For this review, take the finished solid that the model builds, in its own axes (mm). Coordinates: 2 decimals unless noted, no trailing zeros. Loops run counter-clockwise (first coordinate to the right, second up) from the corner with the lowest first, then second, coordinate; pieces in that order, holes last. Notation, with made-up numbers: (-21, 40.5) - (19, 40.5) arc R23 ccw to (19, 59.5) - close; hole circle Ø5 at (27.25, -7.75). An arc over 180 degrees is marked (long way). One line per item, written item: value. Start each with the question number.
1. Take a section at B-B, the plane y = 645.5. State the section outline as (x, z) points, and give its area (3 significant figures).
2. Take a section at A-A, the plane x = 1089.5. State the section outline as (y, z) points, and give its area (3 significant figures).
3. To check wall thickness, follow line 1 (Y direction, x = 1092.5, z = 1.15); line 2 (Y direction, x = 1080.5, z = 0.65); line 3 (X direction, y = 657, z = 0.2). State the ranges of each line that lie inside material, in increasing order. Write a range as from..to.
4. Insertion check: pin 1 (1 mm diameter, centred on x = 1094, z = 0.5, fed in from -Y); pin 2 (0.6 mm diameter, centred on x = 1091.5, z = 1, fed in from -Y); pin 3 (0.6 mm diameter, centred on y = 678, z = 1.5, fed in from +X). Each pin has a flat end and moves straight along its axis. Give the tip position at first contact, or say it passes through.
```python
from build123d import *

# Parameters (mm, degrees)
EXTRUDE_1_DEPTH = 2


with BuildPart() as part:
    # Model → 凸台-拉伸1 (new body)
    with BuildSketch(Plane.XY):
        Polygon((1047.912570376, 680.457705055), (1047.912570376, 676.068532902), (1052.912570376, 676.068532902), (1052.912570376, 671.068532902), (1047.912570376, 671.068532902), (1047.912570376, 668.573157352), (1045.412570376, 668.573157352), (1045.412570376, 658.573157352), (1047.912570376, 658.573157352), (1047.912570376, 643.128332902), (1046.412570376, 643.128332902), (1046.412570376, 633.128332902), (1047.912570376, 633.128332902), (1047.912570376, 629.068532902), (1052.912570376, 629.068532902), (1052.912570376, 624.068532902), (1057.912570376, 624.068532902), (1057.912570376, 623.068532902), (1067.912570376, 623.068532902), (1067.912570376, 624.068532902), (1072.912570376, 624.068532902), (1072.912570376, 623.068532902), (1082.912570376, 623.068532902), (1082.912570376, 624.068532902), (1087.912570376, 624.068532902), (1087.912570376, 629.068532902), (1092.912570376, 629.068532902), (1092.912570376, 633.128332902), (1094.412570376, 633.128332902), (1094.412570376, 643.128332902), (1092.912570376, 643.128332902), (1092.912570376, 658.573157352), (1095.412570376, 658.573157352), (1095.412570376, 668.573157352), (1092.912570376, 668.573157352), (1092.912570376, 671.068532902), (1087.912570376, 671.068532902), (1087.912570376, 676.068532902), (1092.912570376, 676.068532902), (1092.912570376, 680.457705055), align=None)
        with BuildLine():
            Line((1057.912570376, 668.068532902), (1057.912570376, 673.218532902))
            ThreePointArc((1057.912570376, 673.218532902), (1057.440095607, 674.509527351), (1056.245903709, 675.190559496))
            ThreePointArc((1056.245903709, 675.190559496), (1055.64880776, 675.531075569), (1055.412570376, 676.176572793))
            Line((1055.412570376, 676.176572793), (1055.412570376, 676.867577668))
            ThreePointArc((1055.412570376, 676.867577668), (1055.705463595, 677.57468445), (1056.412570376, 677.867577668))
            Line((1056.412570376, 677.867577668), (1083.912570376, 677.867577668))
            ThreePointArc((1083.912570376, 677.867577668), (1084.619677157, 677.57468445), (1084.912570376, 676.867577668))
            Line((1084.912570376, 676.867577668), (1084.912570376, 676.046960027))
            ThreePointArc((1084.912570376, 676.046960027), (1084.729066957, 675.469609757), (1084.245903709, 675.104150985))
            ThreePointArc((1084.245903709, 675.104150985), (1083.279577214, 674.37323344), (1082.912570376, 673.218532902))
            Line((1082.912570376, 673.218532902), (1082.912570376, 668.068532902))
            ThreePointArc((1082.912570376, 668.068532902), (1083.498356813, 666.65431934), (1084.912570376, 666.068532902))
            Line((1084.912570376, 666.068532902), (1085.912570376, 666.068532902))
            ThreePointArc((1085.912570376, 666.068532902), (1087.326783938, 665.482746464), (1087.912570376, 664.068532902))
            Line((1087.912570376, 664.068532902), (1087.912570376, 636.068532902))
            ThreePointArc((1087.912570376, 636.068532902), (1087.326783938, 634.65431934), (1085.912570376, 634.068532902))
            Line((1085.912570376, 634.068532902), (1084.912570376, 634.068532902))
            ThreePointArc((1084.912570376, 634.068532902), (1083.498356813, 633.482746464), (1082.912570376, 632.068532902))
            Line((1082.912570376, 632.068532902), (1082.912570376, 631.068532902))
            ThreePointArc((1082.912570376, 631.068532902), (1082.326783938, 629.65431934), (1080.912570376, 629.068532902))
            Line((1080.912570376, 629.068532902), (1059.912570376, 629.068532902))
            ThreePointArc((1059.912570376, 629.068532902), (1058.498356813, 629.65431934), (1057.912570376, 631.068532902))
            Line((1057.912570376, 631.068532902), (1057.912570376, 632.068532902))
            ThreePointArc((1057.912570376, 632.068532902), (1057.326783938, 633.482746464), (1055.912570376, 634.068532902))
            Line((1055.912570376, 634.068532902), (1054.912570376, 634.068532902))
            ThreePointArc((1054.912570376, 634.068532902), (1053.498356813, 634.65431934), (1052.912570376, 636.068532902))
            Line((1052.912570376, 636.068532902), (1052.912570376, 664.068532902))
            ThreePointArc((1052.912570376, 664.068532902), (1053.498356813, 665.482746464), (1054.912570376, 666.068532902))
            Line((1054.912570376, 666.068532902), (1055.912570376, 666.068532902))
            ThreePointArc((1055.912570376, 666.068532902), (1057.326783938, 666.65431934), (1057.912570376, 668.068532902))
        make_face(mode=Mode.SUBTRACT)
    extrude(amount=EXTRUDE_1_DEPTH)


solid = part.part
```
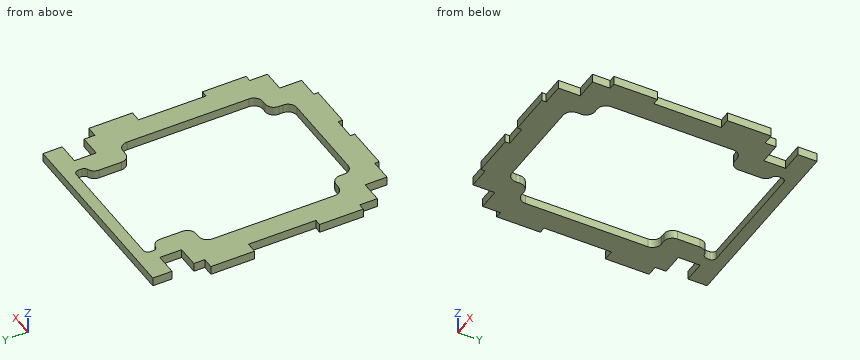
Solutions:
1. outline: (1047.91, 0) - (1052.91, 0) - (1052.91, 2) - (1047.91, 2) - close; (1087.91, 0) - (1092.91, 0) - (1092.91, 2) - (1087.91, 2) - close
1. area: 20.0 mm2
2. outline: (629.07, 0) - (671.07, 0) - (671.07, 2) - (629.07, 2) - close; (676.07, 0) - (680.46, 0) - (680.46, 2) - (676.07, 2) - close
2. area: 92.8 mm2
3. line 1: 629.07..671.07, 676.07..680.46
3. line 2: 623.07..629.07, 677.87..680.46
3. line 3: 1047.91..1052.91, 1087.91..1092.91
4. pin 1: y = 633.13
4. pin 2: y = 629.07
4. pin 3: x = 1092.91
